For this review, take the finished solid that the model builds, in its own axes (mm). A direction names the side the tool comes from. Round coordinates to 2 decimals unless told otherwise and drop trailing zeros. Write each loop counter-clockwise with the first axis right and the second up, starting at its lowest first coordinate (ties: lowest second). Pieces come first, ordered by that corner, then holes. Notation, with made-up numbers: M 58.25,35 L 114.25,35 A35 ccw 114.25,73 Z; hole C 35,24 d8. An arc over 180 degrees is marked long. Answer in a Markdown table with one row per item.
```python
from build123d import *
from build123d.topology import SkipClean

# Parameters (mm, degrees)
SKETCH_1_W          = 47
SKETCH_1_H          = 40
SKETCH_1_R          = 1.5
SKETCH_1_W_2        = 30
SKETCH_1_H_2        = 10
SKETCH_1_H_3        = 55.72
SKETCH_1_W_3        = 15
EXTRUDE_1_DEPTH     = 4
EXTRUDE_START       = 1
SKETCH_3_W          = 8
SKETCH_3_H          = 8
SKETCH_3_R          = 1.5
EXTRUDE_2_DEPTH     = 1
SKETCH_4_R          = 1.5
SKETCH_4_W          = 47
SKETCH_4_H          = 5
CUT_EXTRUDE_2_DEPTH = 4


with BuildPart() as part:
    # 草图1 → 凸台-拉伸1 (new body)
    # profile 1 of 3: a face of its own
    with BuildSketch(Plane(origin=(0, 0, 0), x_dir=(1, 0, 0), z_dir=(0, 1, 0))):
        Rectangle(SKETCH_1_W, SKETCH_1_H)
        with Locations(Location((19.5, -14, 0), (0, 0, 270))):
            Circle(SKETCH_1_R, mode=Mode.SUBTRACT)
        with Locations(Location((19.5, 14, 0), (0, 0, 270))):
            Circle(SKETCH_1_R, mode=Mode.SUBTRACT)
        with Locations(Location((-19.5, -14, 0), (0, 0, 270))):
            Circle(SKETCH_1_R, mode=Mode.SUBTRACT)
        with Locations(Location((-19.5, 14, 0), (0, 0, 270))):
            Circle(SKETCH_1_R, mode=Mode.SUBTRACT)
        with Locations((0, -12)):
            Rectangle(SKETCH_1_W_2, SKETCH_1_H_2, mode=Mode.SUBTRACT)
    # profile 2 of 3: a face of its own
    with BuildSketch(Plane(origin=(0, 0, 0), x_dir=(1, 0, 0), z_dir=(0, 1, 0))):
        with Locations((0, -47.86)):
            Rectangle(SKETCH_1_W, SKETCH_1_H_3)
    # profile 3 of 3: a face of its own
    with BuildSketch(Plane(origin=(0, 0, 0), x_dir=(1, 0, 0), z_dir=(0, 1, 0))):
        with Locations((-7.5, -12)):
            Rectangle(SKETCH_1_W_3, SKETCH_1_H_2)
    extrude(amount=EXTRUDE_1_DEPTH)

    # 草图3 → 凸台-拉伸2 (add)
    # profile 1 of 4: a face of its own
    with SkipClean():  # the faces are left unmerged after this step: merging them gives an invalid solid
        with BuildSketch(Plane.XZ.offset(EXTRUDE_START)):
            with Locations((19.5, -14)):
                Rectangle(SKETCH_3_W, SKETCH_3_H)
            with Locations(Location((19.5, -14, 0), (0, 0, 270))):
                Circle(SKETCH_3_R, mode=Mode.SUBTRACT)
        # profile 2 of 4: a face of its own
        with BuildSketch(Plane.XZ.offset(EXTRUDE_START)):
            with Locations((19.5, 14)):
                Rectangle(SKETCH_3_W, SKETCH_3_H)
            with Locations(Location((19.5, 14, 0), (0, 0, 270))):
                Circle(SKETCH_3_R, mode=Mode.SUBTRACT)
        # profile 3 of 4: a face of its own
        with BuildSketch(Plane.XZ.offset(EXTRUDE_START)):
            with Locations((-19.5, -14)):
                Rectangle(SKETCH_3_W, SKETCH_3_H)
            with Locations(Location((-19.5, -14, 0), (0, 0, 270))):
                Circle(SKETCH_3_R, mode=Mode.SUBTRACT)
        # profile 4 of 4: a face of its own
        with BuildSketch(Plane.XZ.offset(EXTRUDE_START)):
            with Locations((-19.5, 14)):
                Rectangle(SKETCH_3_W, SKETCH_3_H)
            with Locations(Location((-19.5, 14, 0), (0, 0, 270))):
                Circle(SKETCH_3_R, mode=Mode.SUBTRACT)
        extrude(amount=-EXTRUDE_2_DEPTH)

    # 草图4 → 切除-拉伸2 (cut)
    with SkipClean():  # the faces are left unmerged after this step: merging them gives an invalid solid
        with BuildSketch(Plane(origin=(0, 4, 0), x_dir=(1, 0, 0), z_dir=(0, 1, 0))):
            with Locations(Location((9, -30.72, 0), (0, 0, 270))):
                Circle(SKETCH_4_R)
            with Locations(Location((9, -50.72, 0), (0, 0, 270))):
                Circle(SKETCH_4_R)
            with Locations(Location((-9, -50.72, 0), (0, 0, 90))):
                Circle(SKETCH_4_R)
            with Locations(Location((-9, -30.72, 0), (0, 0, 90))):
                Circle(SKETCH_4_R)
            with Locations(Location((-9, -38.72, 0), (0, 0, 90))):
                Circle(SKETCH_4_R)
            with Locations(Location((9, -38.72, 0), (0, 0, 270))):
                Circle(SKETCH_4_R)
            with Locations(Location((9, -58.72, 0), (0, 0, 270))):
                Circle(SKETCH_4_R)
            with Locations(Location((-9, -58.72, 0), (0, 0, 90))):
                Circle(SKETCH_4_R)
            with Locations((0, -73.22)):
                Rectangle(SKETCH_4_W, SKETCH_4_H)
        extrude(amount=-CUT_EXTRUDE_2_DEPTH, mode=Mode.SUBTRACT)


solid = part.part
```
Q1. Mouldability with a two-part tool opening along Z and no side actions: class faces 1 (the face through (8.09, 2.03, 49.53)), 2 (the face through (0, 4, 25)), 3 (the face through (0, 2, -20)), 4 (the face through (-8.425, 2.028, 29.334)) as +Z half, -Z half, draft (parallel to the pull), parting line (faces both ways), or undercut.
Found:
| item | result |
|---|---|
| face 1 | undercut |
| face 2 | draft |
| face 3 | -Z half |
| face 4 | undercut |
Q2. Insertion check: P1, Ø2.5, axis at x = 9, z = 50.72, coming from the +Y side; P2, Ø3.5, axis at x = 9, z = 38.72, coming from the -Y side; P3, Ø3.5, axis at x = -9, z = 58.72, coming from the +Y side; P4, Ø0.8, axis at x = 18, y = -0.5, coming from the +Z side. Each pin has a flat end and moves straight along its axis. Give the tip position at first contact, or say it passes through.
Found:
| item | result |
|---|---|
| P1 | through |
| P2 | y = 0 |
| P3 | y = 4 |
| P4 | z = 18 |
Q3. Take a section at A-A (x = 9). State the section outline as (y, z) points.
Found:
| item | result |
|---|---|
| outline | M 0,-20 L 4,-20 L 4,7 L 0,7 Z; M 0,17 L 4,17 L 4,29.22 L 0,29.22 Z; M 0,32.22 L 4,32.22 L 4,37.22 L 0,37.22 Z; M 0,40.22 L 4,40.22 L 4,49.22 L 0,49.22 Z; M 0,52.22 L 4,52.22 L 4,57.22 L 0,57.22 Z; M 0,60.22 L 4,60.22 L 4,70.72 L 0,70.72 Z |
Q4. Machinability: for faces 5 (the face through (7, 2, 17)), 6 (the face through (-17.8, -1, -13.9)), which of the approach directions +Z, -Z, +X, -X, +Y, -Y give a long, thin tool a straight path to every point of the face, cutting with its end or side? Answer none if there is none.
Found:
| item | result |
|---|---|
| face 5 | +Y, -Y |
| face 6 | +Z, -Z, +X, -X, -Y |
Q5. Take a section at D-D (y = 1.3). State how many separate pieces and enclosed holes the cut face has, then the cut area to 3 significant figures.
Found:
| item | result |
|---|---|
| separate pieces | 1 |
| enclosed holes | 13 |
| area | 4,030 mm² |
Q6. For probe 1 along X at (y, z) = (2.25, 58.72); probe 2 along X at (y, z) = (1.8, -14); probe 3 along Z at (x, y) = (-19, 2.1), list the stretches that pass through material, from the lowest coordinate up.
Found:
| item | result |
|---|---|
| probe 1 | -23.5 to -10.5, -7.5 to 7.5, 10.5 to 23.5 |
| probe 2 | -23.5 to -21, -18 to 18, 21 to 23.5 |
| probe 3 | -20 to -15.41, -12.59 to 12.59, 15.41 to 70.72 |
Q7. Take a section at B-B (x = -9). State the section outline as (y, z) points, then the cut area to 3 significant figures.
Found:
| item | result |
|---|---|
| outline | M 0,-20 L 4,-20 L 4,29.22 L 0,29.22 Z; M 0,32.22 L 4,32.22 L 4,37.22 L 0,37.22 Z; M 0,40.22 L 4,40.22 L 4,49.22 L 0,49.22 Z; M 0,52.22 L 4,52.22 L 4,57.22 L 0,57.22 Z; M 0,60.22 L 4,60.22 L 4,70.72 L 0,70.72 Z |
| area | 315 mm² |
